The model under review builds one solid part; all positions refer to its coordinate system, in mm. A direction names the side the tool comes from. Round coordinates to 2 decimals unless told otherwise and drop trailing zeros. Order: outer loops, then holes, each group sorted by start corner. A loop starts at its lowest first (then second) coordinate and runs counter-clockwise, first axis right, second up. Notation, with made-up numbers: (28.25, 83.25) - (34.25, 83.25) arc R17 ccw to (34.25, 109.25) - close; hole circle Ø8 at (-28.75, 77). An arc over 180 degrees is marked (long way). One line per question, with ' | ' between items. Start each with the question number.
Item 1: Draft analysis for pull direction X (two halves, no side actions). For faces 4 (the face through (-129.1, 0.8, -0.4)), 5 (the face through (-10, -76, 0)), 6 (the face through (-123.5, 1, -3)), state which applies: +X half, -X half, draft (parallel to the pull), parting line (faces both ways), or undercut.
Item 2: Add section A-A on z = -21.5. State the section outline as (x, y) points, and give its area (3 significant figures).
Item 3: Insertion check: pin 1 Ø3.5 at (x, z) = (10, -5) entering from +Y; pin 2 Ø1.5 at (x, z) = (-52.5, -9.5) entering from -Y; pin 3 Ø8 at (x, y) = (48, 24) entering from +Z. Each pin has a flat end and moves straight along its axis. Give the tip position at first contact, or say it passes through.
Item 4: Add section B-B on x = 77.5. State the section outline as (y, z) points, and give its area (3 significant figures).
Item 5: Tool access review of faces 1 (the face through (120, 93, -27)), 2 (the face through (113, 92.5, -14)), 3 (the face through (2, 74.5, -3)): name each direction out of +Z, -Z, +X, -X, +Y, -Y from which nothing blocks a thin tool from reaching the whole face with its end or side.
Item 6: For L1, parallel to X at y = -44, z = -6; L2, parallel to Y at x = -113, z = -11; L3, parallel to X at y = 26, z = -7.75, list the stretches that pass through material, from the lowest coordinate up. Write a range as [from, to].
Item 7: Add section C-C on y = -43.5. State the section outline as (x, z) points.
Item 8: Add section D-D on y = 81. State the section outline as (x, z) points, and give its area (3 significant figures).
from build123d import *

# Parameters (mm, degrees)
F1_DEPTH = 27
F0_W     = 251
F0_H     = 153
F2_DEPTH = 2
F0_W_2   = 198.2
F0_H_2   = 2
F0_W_3   = 2
F0_H_3   = 148.2
F3_DEPTH = 2
F4_DEPTH = 9
F5_DEPTH = 7


with BuildPart() as f1:
    # F0 (on Top) → F1 (new body)
    with BuildSketch(Plane.XY):
        Polygon((99.1, 94.5), (99.1, 92.5), (127.1, 92.5), (127.1, 74.5), (129.1, 74.5), (129.1, 94.5), align=None)
        Polygon((129.1, -73.7), (127.1, -73.673005), (127.1, -91.7), (99.1, -91.7), (99.1, -93.7), (129.1, -93.7), align=None)
        Polygon((-127.1, -91.7), (-127.1, -73.7), (-129.1, -73.7), (-129.1, -93.7), (-99.1, -93.7), (-99.1, -91.7), align=None)
        Polygon((-127.1, 74.5), (-127.1, 92.5), (-99.1, 92.5), (-99.1, 94.5), (-129.1, 94.5), (-129.1, 74.5), align=None)
    extrude(amount=-F1_DEPTH)

    # F0 (on Top) → F2 (join)
    with BuildSketch(Plane.XY):
        Polygon((-99.1, 92.5), (-127.1, 92.5), (-127.1, 74.5), (-127.1, -73.7), (-127.1, -91.7), (-99.1, -91.7), (99.1, -91.7), (127.1, -91.7), (127.1, -73.673005), (127.1, 74.5), (127.1, 92.5), (99.1, 92.5), align=None)
        Rectangle(F0_W, F0_H, mode=Mode.SUBTRACT)
        Rectangle(F0_W, F0_H)
        with BuildLine():
            ThreePointArc((-123.5, 64.5), (-120.571068, 71.571068), (-113.5, 74.5))
            Line((-113.5, 74.5), (113.5, 74.5))
            ThreePointArc((113.5, 74.5), (120.571068, 71.571068), (123.5, 64.5))
            Line((123.5, 64.5), (123.5, -64.5))
            ThreePointArc((123.5, -64.5), (120.571068, -71.571068), (113.5, -74.5))
            Line((113.5, -74.5), (-113.5, -74.5))
            ThreePointArc((-113.5, -74.5), (-120.571068, -71.571068), (-123.5, -64.5))
            Line((-123.5, -64.5), (-123.5, 64.5))
        make_face(mode=Mode.SUBTRACT)
    extrude(amount=-F2_DEPTH)

    # F0 (on Top) → F3 (join)
    with BuildSketch(Plane.XY):
        with Locations((0, -92.7)):
            Rectangle(F0_W_2, F0_H_2)
        with Locations((0, 93.5)):
            Rectangle(F0_W_2, F0_H_2)
        with Locations((-128.1, 0.4)):
            Rectangle(F0_W_3, F0_H_3)
        Polygon((129.1, 74.5), (127.1, 74.5), (127.1, -73.673005), (129.1, -73.7), align=None)
    extrude(amount=-F3_DEPTH)

    # F0 (on Top) → F4 (join)
    with BuildSketch(Plane.XY):
        Rectangle(F0_W, F0_H)
        with BuildLine():
            ThreePointArc((-123.5, 64.5), (-120.571068, 71.571068), (-113.5, 74.5))
            Line((-113.5, 74.5), (113.5, 74.5))
            ThreePointArc((113.5, 74.5), (120.571068, 71.571068), (123.5, 64.5))
            Line((123.5, 64.5), (123.5, -64.5))
            ThreePointArc((123.5, -64.5), (120.571068, -71.571068), (113.5, -74.5))
            Line((113.5, -74.5), (-113.5, -74.5))
            ThreePointArc((-113.5, -74.5), (-120.571068, -71.571068), (-123.5, -64.5))
            Line((-123.5, -64.5), (-123.5, 64.5))
        make_face(mode=Mode.SUBTRACT)
        with BuildLine():
            Line((113.5, 74.5), (-113.5, 74.5))
            ThreePointArc((-113.5, 74.5), (-120.571068, 71.571068), (-123.5, 64.5))
            Line((-123.5, 64.5), (-123.5, -64.5))
            ThreePointArc((-123.5, -64.5), (-120.571068, -71.571068), (-113.5, -74.5))
            Line((-113.5, -74.5), (113.5, -74.5))
            ThreePointArc((113.5, -74.5), (120.571068, -71.571068), (123.5, -64.5))
            Line((123.5, -64.5), (123.5, 64.5))
            ThreePointArc((123.5, 64.5), (120.571068, 71.571068), (113.5, 74.5))
        make_face()
    extrude(amount=-F4_DEPTH)

    # F0 (on Top) → F5 (cut)
    with BuildSketch(Plane.XY):
        with BuildLine():
            Line((113.5, 74.5), (-113.5, 74.5))
            ThreePointArc((-113.5, 74.5), (-120.571068, 71.571068), (-123.5, 64.5))
            Line((-123.5, 64.5), (-123.5, -64.5))
            ThreePointArc((-123.5, -64.5), (-120.571068, -71.571068), (-113.5, -74.5))
            Line((-113.5, -74.5), (113.5, -74.5))
            ThreePointArc((113.5, -74.5), (120.571068, -71.571068), (123.5, -64.5))
            Line((123.5, -64.5), (123.5, 64.5))
            ThreePointArc((123.5, 64.5), (120.571068, 71.571068), (113.5, 74.5))
        make_face()
    extrude(amount=-F5_DEPTH, mode=Mode.SUBTRACT)


solid = f1.part
Determined:
1) face 4: -X half | face 5: draft | face 6: undercut
2) outline: (-129.1, -93.7) - (-99.1, -93.7) - (-99.1, -91.7) - (-127.1, -91.7) - (-127.1, -73.7) - (-129.1, -73.7) - close; (-129.1, 74.5) - (-127.1, 74.5) - (-127.1, 92.5) - (-99.1, 92.5) - (-99.1, 94.5) - (-129.1, 94.5) - close; (99.1, -93.7) - (129.1, -93.7) - (129.1, -73.7) - (127.1, -73.67) - (127.1, -91.7) - (99.1, -91.7) - close; (99.1, 92.5) - (127.1, 92.5) - (127.1, 74.5) - (129.1, 74.5) - (129.1, 94.5) - (99.1, 94.5) - close | area: 384 mm2
3) pin 1: y = 76.5 | pin 2: y = -76.5 | pin 3: z = -7
4) outline: (-93.7, -2) - (-76.5, -2) - (-76.5, -9) - (76.5, -9) - (76.5, -2) - (94.5, -2) - (94.5, 0) - (74.5, 0) - (74.5, -7) - (-74.5, -7) - (-74.5, 0) - (-93.7, 0) - close | area: 404 mm2
5) face 1: -Z, +X, -X, +Y, -Y | face 2: -Z | face 3: +Z
6) L1: [-125.5, -123.5], [123.5, 125.5] | L2: [-93.7, -91.7], [92.5, 94.5] | L3: [-125.5, 125.5]
7) outline: (-129.1, -2) - (-125.5, -2) - (-125.5, -9) - (125.5, -9) - (125.5, -2) - (129.1, -2) - (129.1, 0) - (123.5, 0) - (123.5, -7) - (-123.5, -7) - (-123.5, 0) - (-129.1, 0) - close
8) outline: (-129.1, -27) - (-127.1, -27) - (-127.1, -2) - (127.1, -2) - (127.1, -27) - (129.1, -27) - (129.1, 0) - (-129.1, 0) - close | area: 616 mm2
